Work out the finished part from the listing and answer in its coordinate system (mm). Face numbers are marked on the shaded views. Round coordinates to 2 decimals unless told otherwise and drop trailing zeros. Write each loop counter-clockwise with the first axis right and the second up, starting at its lowest first coordinate (ties: lowest second). Pieces come first, ordered by that corner, then holes. Notation, with made-up numbers: (25.25, 48) - (74.25, 48) arc R25 cw to (74.25, 67) - close; hole circle Ø1 at (-28, 57). An arc over 180 degrees is marked (long way). Write item = value, one per line. Start each with the question number.
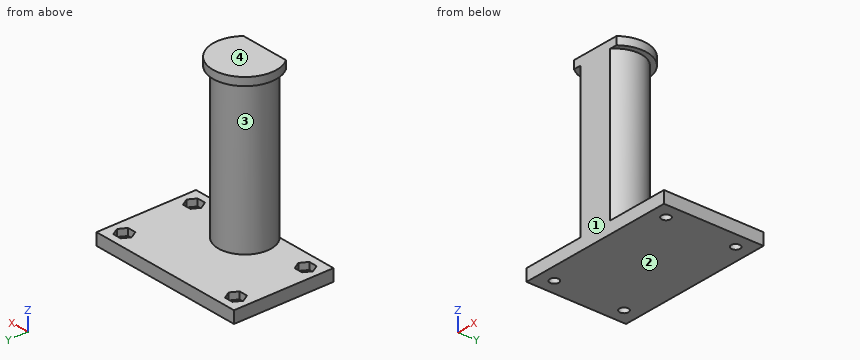
Autodesk Inventor part; units mm, degrees
ref_plane "Work Plane1" through (0, 0, 26) normal (0, 0, 1) x (1, 0, 0)
ref_plane "Work Plane2" through (0, 0, 61) normal (0, 0, 1) x (1, 0, 0)
ref_plane "YZ Plane" through (0, 0, 0) normal (1, 0, 0) x (0, 1, 0)
sketch "Sketch1" plane through (0, 0, 0) normal (0, 0, 1) x (1, 0, 0)
  line L0 (0, 0) -> (80, 0)
  line L1 (80, 0) -> (80, 50)
  line L2 (80, 50) -> (0, 50)
  line L3 (0, 50) -> (0, 0)
  dimension "d0" = 80
  dimension "d1" = 50
extrude "Extrusion1" add sketch "Sketch1" along normal blind 6
sketch "Sketch2" plane through (0, 0, 6) normal (0, 0, 1) x (1, 0, 0)
  line L0 (80, 50) -> (0, 50)
  line L1 (0, 50) -> (0, 0)
  arc A0 (48.6927, 0) -> (31.3073, 0) centre (40, 10) ccw
  line L2 (31.3073, 0) -> (48.6927, 0)
  dimension "d11" = 26.5
  dimension "d12" = 40
  dimension "d13" = 40
  dimension "d14" = 10
extrude "Extrusion2" add sketch "Sketch2" along normal blind 75
sketch "Sketch8" plane through (0, 0, 81) normal (0, 0, 1) x (1, 0, 0)
  arc A0 (48.6927, 0) -> (31.3073, 0) centre (40, 10) ccw
  line L0 (31.3073, 0) -> (48.6927, 0)
  arc A1 (52.3616, 0) -> (27.6384, 0) centre (40, 10) ccw
  line L1 (31.3073, 0) -> (27.6384, 0)
  line L2 (48.6927, 0) -> (52.3616, 0)
  point P0 (0, 0)
  dimension "d30" = 31.8
extrude "Extrusion7" add sketch "Sketch8" along normal blind 4
sketch "Sketch9" plane through (0, 0, 0) normal (0, 0, -1) x (-1, 0, 0)
  line L0 (0, 0) -> (-80, 0)
  line L1 (-80, 0) -> (-80, 50)
  point P0 (-72.5, 42.5)
  point P1 (-72.5, 7.5)
  point P2 (-7.5, 42.5)
  point P3 (-7.5, 7.5)
  dimension "d33" = 65
  dimension "d34" = 35
  dimension "d35" = 7.5
  dimension "d36" = 7.5
hole "Hole1" at (72.5, 42.5, 0) at (72.5, 7.5, 0) at (7.5, 42.5, 0) at (7.5, 7.5, 0) direction (0, 0, 1) diameter 4.5 end through all
sketch "Sketch10" plane through (0, 0, 6) normal (0, 0, 1) x (1, 0, 0)
  circle A0 centre (7.5, 42.5) radius 2.25
  circle A1 centre (72.5, 42.5) radius 2.25
  circle A2 centre (72.5, 7.5) radius 2.25
  circle A3 centre (7.5, 7.5) radius 2.25
  line L0 (11.7724, 42.5) -> (9.6362, 38.8)
  line L1 (9.6362, 38.8) -> (5.3638, 38.8)
  line L2 (5.3638, 38.8) -> (3.2276, 42.5)
  line L3 (3.2276, 42.5) -> (5.3638, 46.2)
  line L4 (5.3638, 46.2) -> (9.6362, 46.2)
  line L5 (9.6362, 46.2) -> (11.7724, 42.5)
  line L6 (11.7724, 7.5) -> (9.6362, 3.8)
  line L7 (9.6362, 3.8) -> (5.3638, 3.8)
  line L8 (5.3638, 3.8) -> (3.2276, 7.5)
  line L9 (3.2276, 7.5) -> (5.3638, 11.2)
  line L10 (5.3638, 11.2) -> (9.6362, 11.2)
  line L11 (9.6362, 11.2) -> (11.7724, 7.5)
  line L12 (76.7724, 7.5) -> (74.6362, 3.8)
  line L13 (74.6362, 3.8) -> (70.3638, 3.8)
  line L14 (70.3638, 3.8) -> (68.2276, 7.5)
  line L15 (68.2276, 7.5) -> (70.3638, 11.2)
  line L16 (70.3638, 11.2) -> (74.6362, 11.2)
  line L17 (74.6362, 11.2) -> (76.7724, 7.5)
  line L18 (76.7724, 42.5) -> (74.6362, 38.8)
  line L19 (74.6362, 38.8) -> (70.3638, 38.8)
  line L20 (70.3638, 38.8) -> (68.2276, 42.5)
  line L21 (68.2276, 42.5) -> (70.3638, 46.2)
  line L22 (70.3638, 46.2) -> (74.6362, 46.2)
  line L23 (74.6362, 46.2) -> (76.7724, 42.5)
  dimension "d44" = 7.4
extrude "Extrusion8" cut sketch "Sketch10" against normal blind 3.5
sketch "Sketch4" plane through (0, 0, 26) normal (0, 0, 1) x (1, 0, 0)
  arc A0 (62.9129, 0) -> (17.0871, 0) centre (40, 10) ccw
  line L0 (17.0871, 0) -> (62.9129, 0)
  circle A1 centre (40, 24.5) radius 11 construction
  arc A2 (28, 24.5) -> (52, 24.5) centre (40, 24.5) ccw
  line L1 (28, 24.5) -> (28, 31.9317)
  line L2 (52, 24.5) -> (52, 31.9317)
  arc A3 (62.9129, 0) -> (17.0871, 0) centre (40, 10) ccw
  point P0 (0, 0)
  dimension "d15" = 22
  dimension "d16" = 14.5
  dimension "d17" = 24
sketch "Sketch5" plane through (0, 0, 61) normal (0, 0, 1) x (1, 0, 0)
  arc A0 (62.9129, 0) -> (17.0871, 0) centre (40, 10) ccw
  line L0 (17.0871, 0) -> (62.9129, 0)
  arc A1 (28, 24.5) -> (52, 24.5) centre (40, 24.5) ccw
  line L1 (52, 31.9317) -> (52, 24.5)
  arc A2 (52, 31.9317) -> (28, 31.9317) centre (40, 10) ccw
  line L2 (28, 24.5) -> (28, 31.9317)
  point P0 (0, 0)
sketch "Sketch6" plane through (0, 0, 26) normal (0, 0, 1) x (1, 0, 0)
  arc A0 (28, 24.5) -> (52, 24.5) centre (40, 24.5) ccw
  line L0 (52, 31.9317) -> (52, 24.5)
  arc A1 (52, 31.9317) -> (28, 31.9317) centre (40, 10) ccw
  line L1 (28, 24.5) -> (28, 31.9317)
  arc A2 (35.75, 24.5) -> (44.25, 24.5) centre (40, 24.5) ccw
  line L2 (35.75, 26.9) -> (35.75, 34.6361)
  arc A3 (52, 31.9317) -> (28, 31.9317) centre (40, 10) ccw
  line L3 (44.25, 26.9) -> (44.25, 34.6361)
  arc A4 (35.75, 24.5) -> (35.75, 26.9) centre (34.15, 25.7) ccw
  arc A5 (44.25, 26.9) -> (44.25, 24.5) centre (45.85, 25.7) ccw
  point P0 (0, 0)
  dimension "d23" = 8.5
  dimension "d24" = 2
  dimension "d25" = 1.6
sketch "Sketch7" plane through (0, 0, 61) normal (0, 0, 1) x (1, 0, 0)
  arc A0 (35.75, 24.5) -> (44.25, 24.5) centre (40, 24.5) ccw
  arc A1 (44.25, 26.9) -> (44.25, 24.5) centre (45.85, 25.7) ccw
  line L0 (44.25, 34.6361) -> (44.25, 26.9)
  arc A2 (44.25, 34.6361) -> (35.75, 34.6361) centre (40, 10) ccw
  line L1 (35.75, 26.9) -> (35.75, 34.6361)
  arc A3 (35.75, 24.5) -> (35.75, 26.9) centre (34.15, 25.7) ccw
  point P0 (0, 0)
properties part number "SpoolHolderSingleHatchbox" material "ABS Plastic"
1. Find section C-C on x = 57. Give the vertices of the cut face in (y, z).
2. Find section D-D on z = 37. Give the vertices of the cut face in (x, y), plus the area to 3 significant figures.
3. Each of these flat-tipped pins is pushed along its axis until it touches: pin 1 (2 mm diameter, centred on x = 71.5, y = 14.5, fed in from +Z); pin 2 (6 mm diameter, centred on x = 41.5, z = 74, fed in from +Y); pin 3 (2 mm diameter, centred on x = 31.5, y = 24.5, fed in from -Z); pin 4 (4 mm diameter, centred on x = 7.5, y = 42.5, fed in from -Z). Where does it stop, or does it pass through?
4. Consider line 1 (Y direction, x = 72.5, z = 0.9); line 2 (X direction, y = 42.5, z = 2.05); line 3 (Z direction, x = 43, y = 46). Determine where each line is inside the solid, lowest interval first.
5. For a pull along Z with two mould halves and no side action, classify the marked faces 1, 2, 3 and 4 as released by +Z, released by -Z, zero draft, split by the parting line, or undercut.
6. Find section A-A on x = 7.5. Give the vertices of the cut face in (y, z).
7. Find section B-B on y = 19. Give the vertices of the cut face in (x, z).
Answer key:
q1.outline = (0, 0) - (50, 0) - (50, 6) - (0, 6) - close
q2.outline = (31.31, 0) - (48.69, 0) arc R13.25 ccw (long way) to start
q2.area = 513 mm²
q3.pin_1 = 6
q3.pin_2 = 23.25
q3.pin_3 = 0
q3.pin_4 = through
q4.line_1 = 0 to 5.25, 9.75 to 40.25, 44.75 to 50
q4.line_2 = 0 to 5.25, 9.75 to 70.25, 74.75 to 80
q4.line_3 = 0 to 6
q5.face_1 = zero draft
q5.face_2 = released by -Z
q5.face_3 = undercut
q5.face_4 = released by +Z
q6.outline = (0, 0) - (5.25, 0) - (5.25, 2.5) - (3.8, 2.5) - (3.8, 6) - (0, 6) - close; (9.75, 0) - (40.25, 0) - (40.25, 2.5) - (38.8, 2.5) - (38.8, 6) - (11.2, 6) - (11.2, 2.5) - (9.75, 2.5) - close; (44.75, 0) - (50, 0) - (50, 6) - (46.2, 6) - (46.2, 2.5) - (44.75, 2.5) - close
q7.outline = (0, 0) - (80, 0) - (80, 6) - (49.72, 6) - (49.72, 81) - (53.11, 81) - (53.11, 85) - (26.89, 85) - (26.89, 81) - (30.28, 81) - (30.28, 6) - (0, 6) - close
